Design review of the part built by this model. Coordinates are the model's own, in mm. Give positions to 0.01 mm unless a question says otherwise; leave off trailing zeros. Write each loop counter-clockwise with the first axis right and the second up, starting at its lowest first coordinate (ties: lowest second). Pieces come first, ordered by that corner, then holes.
```python
from build123d import *

# Parameters (mm, degrees)
F0_R     = 11.43
F1_DEPTH = 50.8
F2_R     = 11.43
F4_D     = 4.318
F4_DEPTH = 11.431


with BuildPart() as f1:
    # F0 (on Front) → F1 (new body, symmetric)
    with BuildSketch(Plane.XZ):
        Circle(F0_R)
    extrude(amount=F1_DEPTH, both=True)

    # F2
    f2_edges = [f1.edges().sort_by_distance(p)[0] for p in [
        (-11.43, 50.8, 0),
        (-11.43, -50.8, 0),
    ]]
    fillet(f2_edges, radius=F2_R)

    # F4 (through all, one way)
    with BuildSketch(Plane.YZ):
        with Locations((0, 0)):
            Circle(F4_D / 2)
    extrude(amount=-F4_DEPTH, mode=Mode.SUBTRACT)


solid = f1.part
```
(1) Mouldability with a two-part tool opening along Y and no side actions: class faces 1 (the face through (-5.63, -0.28, 2.14)), 2 (the face through (10.902, -0.551, 3.433)), 3 (the face through (0, 0, 0)) as pulls with the +Y half, pulls with the -Y half, needs draft (parallel to the pull), parting line crosses it, or undercut.
Resolved:
face 1: undercut
face 2: needs draft
face 3: undercut
(2) Consider section A-A, the plane z = 0. Give the boundary of the cut face in (x, y), then the cut area to 3 significant figures.
Resolved:
outline: (-11.43, -39.37) arc R11.43 ccw to (11.43, -39.37) - (11.43, 39.37) arc R11.43 ccw to (-11.43, 39.37) - (-11.43, 2.16) - (0, 2.16) - (0, -2.16) - (-11.43, -2.16) - close
area: 2,160 mm2
(3) Clearance check with flat-ended pins moving along their axes: P1, Ø2, axis at y = 27, z = 7, coming from the -X side; P2, Ø1.5, axis at y = 37.5, z = -3, coming from the +X side; P3, Ø4, axis at x = 3.5, z = -8, coming from the +Y side. State where each tip first meets the part, or that it passes through.
Resolved:
P1: stops at x = -9.73
P2: stops at x = 11.21
P3: stops at y = 48.61
(4) Consider section D-D, the plane x = 4.5. Give the boundary of the cut face in (y, z).
Resolved:
outline: (-39.37, -10.51) - (39.37, -10.51) arc R10.51 ccw to (39.37, 10.51) - (-39.37, 10.51) arc R10.51 ccw to start
(5) To check wall thickness, follow L1, parallel to Z at x = -0.25, y = 0; L2, parallel to Y at x = -3.5, z = 0; L3, parallel to Z at x = -3.75, y = 0. State the ranges of each line that lie inside material, in increasing order.
Resolved:
L1: z = -11.43 to -2.16, 2.16 to 11.43
L2: y = -50.25 to -2.16, 2.16 to 50.25
L3: z = -10.8 to -2.16, 2.16 to 10.8
(6) Consider section C-C, the plane y = -22.5. Give the boundary of the cut face in (x, z).
Resolved:
outline: circle Ø22.86 at (0, 0)
(7) Consider section B-B, the plane x = -5.75. Give the boundary of the cut face in (y, z).
Resolved:
outline: (-39.37, -9.88) - (39.37, -9.88) arc R9.88 ccw to (39.37, 9.88) - (-39.37, 9.88) arc R9.88 ccw to start; hole circle Ø4.32 at (0, 0)
